from build123d import *

# Parameters (mm, degrees)
F0_R     = 7
F1_DEPTH = 0.4
F3_DEPTH = 14
F5_W     = 4
F5_H     = 2.4
F6_DEPTH = 0.4


with BuildPart() as f1:
    # F0 (on Front) → F1 (new body)
    with BuildSketch(Plane.XZ):
        with BuildLine():
            Line((-17.5, -27.5), (17.5, -27.5))
            ThreePointArc((17.5, -27.5), (24.571068, -24.571068), (27.5, -17.5))
            Line((27.5, -17.5), (27.5, 17.5))
            ThreePointArc((27.5, 17.5), (24.571068, 24.571068), (17.5, 27.5))
            Line((17.5, 27.5), (-17.5, 27.5))
            ThreePointArc((-17.5, 27.5), (-24.571068, 24.571068), (-27.5, 17.5))
            Line((-27.5, 17.5), (-27.5, -17.5))
            ThreePointArc((-27.5, -17.5), (-24.571068, -24.571068), (-17.5, -27.5))
        make_face()
        Circle(F0_R, mode=Mode.SUBTRACT)
    extrude(amount=F1_DEPTH)

    # F2 (on Front) → F3 (join)
    with BuildSketch(Plane.XZ):
        with BuildLine():
            ThreePointArc((27.9, 17.5), (24.853911, 24.853911), (17.5, 27.9))
            Line((17.5, 27.9), (-17.5, 27.9))
            ThreePointArc((-17.5, 27.9), (-24.853911, 24.853911), (-27.9, 17.5))
            Line((-27.9, 17.5), (-27.9, -17.5))
            ThreePointArc((-27.9, -17.5), (-24.853911, -24.853911), (-17.5, -27.9))
            Line((-17.5, -27.9), (17.5, -27.9))
            ThreePointArc((17.5, -27.9), (24.853911, -24.853911), (27.9, -17.5))
            Line((27.9, -17.5), (27.9, 17.5))
        make_face()
        with BuildLine():
            ThreePointArc((27.5, -17.5), (24.571068, -24.571068), (17.5, -27.5))
            Line((17.5, -27.5), (-17.5, -27.5))
            ThreePointArc((-17.5, -27.5), (-24.571068, -24.571068), (-27.5, -17.5))
            Line((-27.5, -17.5), (-27.5, 17.5))
            ThreePointArc((-27.5, 17.5), (-24.571068, 24.571068), (-17.5, 27.5))
            Line((-17.5, 27.5), (17.5, 27.5))
            ThreePointArc((17.5, 27.5), (24.571068, 24.571068), (27.5, 17.5))
            Line((27.5, 17.5), (27.5, -17.5))
        make_face(mode=Mode.SUBTRACT)
    extrude(amount=F3_DEPTH)

    # F5 (on face) → F6 (join)
    with BuildSketch(Plane(origin=(0, -14, 0), x_dir=(-1, 0, 0), z_dir=(0, 1, 0))):
        with Locations((-15.5, -26.7)):
            Rectangle(F5_W, F5_H)
        with Locations((15.5, -26.7)):
            Rectangle(F5_W, F5_H)
        with Locations((15.5, 26.7)):
            Rectangle(F5_W, F5_H)
        with Locations((-15.5, 26.7)):
            Rectangle(F5_W, F5_H)
    extrude(amount=F6_DEPTH)


solid = f1.part
Work out the finished part from the listing and answer in its coordinate system (mm). A direction names the side the tool comes from. Coordinates: 2 decimals unless noted, no trailing zeros. Order: outer loops, then holes, each group sorted by start corner. A loop starts at its lowest first (then second) coordinate and runs counter-clockwise, first axis right, second up. Notation, with made-up numbers: (66.5, 36) - (91.5, 36) arc R30 ccw to (91.5, 60) - close; hole circle Ø8 at (10, 64.5). An arc over 180 degrees is marked (long way). Put each result on its own line as item: value. Start each with the question number.
1) Find section D-D (z = 8). Give the vertices of the cut face in (x, y), plus the area to 3 significant figures.
2) Find the intervals of material crossed by line 1 (X direction, y = -1, z = -3); line 2 (Z direction, x = 0, y = -0.15), in increasing order. Write a range as from..to.
3) For faces 4 (the flat face through (16, -13.6, 27)), 5 (the cylindrical face through (24.773, -6.902, -24.934)), 6 (the cylindrical face through (24.49, -7.1, 24.65)), determine the directions among +Z, -Z, +X, -X, +Y, -Y from which every point of the face is accessible in a straight line to the end or side of a thin tool.
4) For a pull along Y with two mould halves and no side action, classify faces 1 (the cylindrical face through (-24.65, -7.1, 24.49)), 2 (the flat face through (0, -7, 27.5)), 3 (the flat face through (-15, -14, 27)) as released by +Y, released by -Y, zero draft, split by the parting line, or undercut.
5) Find section A-A (x = 0). Give the vertices of the cut face in (y, z), plus the area to 3 significant figures.
6) Flat-ended cylindrical pins translate along their axes: pin 1 (6 mm diameter, centred on y = -3, z = 21, fed in from +X); pin 2 (2 mm diameter, centred on x = -10.5, z = -9, fed in from -Y); pin 3 (2 mm diameter, centred on x = 19.5, y = -6.5, fed in from +Z). Find the tip coordinate at first contact, or state that the pin passes through.
7) Find section C-C (y = -6.5). Give the vertices of the cut face in (x, z).
8) Find section B-B (z = 0). Give the vertices of the cut face in (x, y), plus the area to 3 significant figures.
Results list:
1. outline: (-27.9, -14) - (-27.5, -14) - (-27.5, -0.4) - (27.5, -0.4) - (27.5, -14) - (27.9, -14) - (27.9, 0) - (-27.9, 0) - close
1. area: 33.2 mm^2
2. line 1: x = -27.9..-27.5, 27.5..27.9
2. line 2: z = -27.9..-7, 7..27.9
3. face 4: none
3. face 5: -Z, +X, +Y, -Y
3. face 6: -Y
4. face 1: zero draft
4. face 2: undercut
4. face 3: released by -Y
5. outline: (-14, -27.9) - (0, -27.9) - (0, -7) - (-0.4, -7) - (-0.4, -27.5) - (-14, -27.5) - close; (-14, 27.5) - (-0.4, 27.5) - (-0.4, 7) - (0, 7) - (0, 27.9) - (-14, 27.9) - close
5. area: 27.6 mm^2
6. pin 1: stops at x = 27.89
6. pin 2: stops at y = -0.4
6. pin 3: stops at z = 27.85
7. outline: (-27.9, -17.5) arc R10.4 ccw to (-17.5, -27.9) - (17.5, -27.9) arc R10.4 ccw to (27.9, -17.5) - (27.9, 17.5) arc R10.4 ccw to (17.5, 27.9) - (-17.5, 27.9) arc R10.4 ccw to (-27.9, 17.5) - close; hole (-27.5, -17.5) arc R10 ccw to (-17.5, -27.5) - (17.5, -27.5) arc R10 ccw to (27.5, -17.5) - (27.5, 17.5) arc R10 ccw to (17.5, 27.5) - (-17.5, 27.5) arc R10 ccw to (-27.5, 17.5) - close
8. outline: (-27.9, -14) - (-27.5, -14) - (-27.5, -0.4) - (-7, -0.4) - (-7, 0) - (-27.9, 0) - close; (7, -0.4) - (27.5, -0.4) - (27.5, -14) - (27.9, -14) - (27.9, 0) - (7, 0) - close
8. area: 27.6 mm^2
